The listing builds one solid part. Answer for the finished solid, in the listing's coordinates (mm). A direction names the side the tool comes from. Coordinates: 2 decimals unless noted, no trailing zeros. Order: outer loops, then holes, each group sorted by start corner. A loop starts at its lowest first (then second) coordinate and runs counter-clockwise, first axis right, second up.
```python
from build123d import *

# Parameters (mm, degrees)
CROQUIS1_W              = 20
CROQUIS1_H              = 2.5
SALIENTE_EXTRUIR1_DEPTH = 3
CROQUIS2_R              = 0.45
SALIENTE_EXTRUIR2_DEPTH = 3
CROQUIS3_R              = 0.45
SALIENTE_EXTRUIR3_DEPTH = 9


with BuildPart() as part:
    # Croquis1 → Saliente-Extruir1 (new body)
    with BuildSketch(Plane.XY):
        Rectangle(CROQUIS1_W, CROQUIS1_H)
    extrude(amount=SALIENTE_EXTRUIR1_DEPTH)

    # Croquis2 → Saliente-Extruir2 (add)
    with BuildSketch(Plane(origin=(0, 1.25, 0), x_dir=(1, 0, 0), z_dir=(0, 1, 0))):
        with Locations((-8.75, -1.5)):
            Circle(CROQUIS2_R)
        with Locations((-6.25, -1.5)):
            Circle(CROQUIS2_R)
        with Locations((-3.75, -1.5)):
            Circle(CROQUIS2_R)
        with Locations((-1.25, -1.5)):
            Circle(CROQUIS2_R)
        with Locations((1.25, -1.5)):
            Circle(CROQUIS2_R)
        with Locations((3.75, -1.5)):
            Circle(CROQUIS2_R)
        with Locations((6.25, -1.5)):
            Circle(CROQUIS2_R)
        with Locations((8.75, -1.5)):
            Circle(CROQUIS2_R)
    extrude(amount=SALIENTE_EXTRUIR2_DEPTH)

    # Croquis3 → Saliente-Extruir3 (add)
    with BuildSketch(Plane.XZ.offset(1.25)):
        with Locations((-8.75, 1.5)):
            Circle(CROQUIS3_R)
        with Locations((-6.25, 1.5)):
            Circle(CROQUIS3_R)
        with Locations((-3.75, 1.5)):
            Circle(CROQUIS3_R)
        with Locations((-1.25, 1.5)):
            Circle(CROQUIS3_R)
        with Locations((1.25, 1.5)):
            Circle(CROQUIS3_R)
        with Locations((3.75, 1.5)):
            Circle(CROQUIS3_R)
        with Locations((6.25, 1.5)):
            Circle(CROQUIS3_R)
        with Locations((8.75, 1.5)):
            Circle(CROQUIS3_R)
    extrude(amount=SALIENTE_EXTRUIR3_DEPTH)


solid = part.part
```
1) A cutting plane is placed at C-C, the plane z = 0.2. Write down the section's boundary in (x, y).
2) For faces 4 (the cylindrical face through (4.166, -5.687, 1.328)), 5 (the cylindrical face through (6.666, 2.729, 1.672)), 6 (the flat face through (3.7, 4.25, 1.5)), determine the directions among +Z, -Z, +X, -X, +Y, -Y from which every point of the face is accessible in a straight line to the end or side of a thin tool.
3) A cutting plane is placed at B-B, the plane x = 8.75. Write down the section's boundary in (y, z).
4) A cutting plane is placed at A-A, the plane y = -7.25. Write down the section's boundary in (x, z), plus the area to 3 significant figures.
5) This flat-tipped pin is pushed along its axis until it touches: P1, Ø6, axis at x = 4.5, y = -7.5, coming from the -Z side. Where does it stop, or does it pass through?
6) Straight lines are drawn through the part: probe 1 along Y at (x, z) = (-4, 0.85); probe 2 along Z at (x, y) = (6.25, -8.5). For each, find the intervals that lie inside material, in ascending order.
7) The mould has two halves that part along X. Classify faces 1 (the flat face through (-10, 0, 1)), 2 (the cylindrical face through (1.666, 2.729, 1.672)), 3 (the flat face through (6.2, -10.25, 1.5)): released by +X, released by -X, zero draft, split by the parting line, or undercut.
8) A cutting plane is placed at D-D, the plane x = -9. Write down the section's boundary in (y, z).
Working result:
1. outline: (-10, -1.25) - (10, -1.25) - (10, 1.25) - (-10, 1.25) - close
2. face 4: -Y
2. face 5: +Y
2. face 6: +Z, -Z, +X, -X, +Y
3. outline: (-10.25, 1.05) - (-1.25, 1.05) - (-1.25, 0) - (1.25, 0) - (1.25, 1.05) - (4.25, 1.05) - (4.25, 1.95) - (1.25, 1.95) - (1.25, 3) - (-1.25, 3) - (-1.25, 1.95) - (-10.25, 1.95) - close
4. outline: circle Ø0.9 at (-8.75, 1.5); circle Ø0.9 at (-6.25, 1.5); circle Ø0.9 at (-3.75, 1.5); circle Ø0.9 at (-1.25, 1.5); circle Ø0.9 at (1.25, 1.5); circle Ø0.9 at (3.75, 1.5); circle Ø0.9 at (6.25, 1.5); circle Ø0.9 at (8.75, 1.5)
4. area: 5.09 mm2
5. P1: stops at z = 1.05
6. probe 1: y = -1.25 to 1.25
6. probe 2: z = 1.05 to 1.95
7. face 1: released by -X
7. face 2: undercut
7. face 3: zero draft
8. outline: (-10.25, 1.13) - (-1.25, 1.13) - (-1.25, 0) - (1.25, 0) - (1.25, 1.13) - (4.25, 1.13) - (4.25, 1.87) - (1.25, 1.87) - (1.25, 3) - (-1.25, 3) - (-1.25, 1.87) - (-10.25, 1.87) - close
